Read the model definition and answer for the solid it produces. Units are mm, in the model's axes. Face numbers are marked on the shaded views. A direction names the side the tool comes from. Round coordinates to 2 decimals unless told otherwise and drop trailing zeros. Loops run counter-clockwise (first coordinate to the right, second up) from the corner with the lowest first, then second, coordinate; pieces in that order, holes last. Notation, with made-up numbers: M 89,55.5 L 130,55.5 A19 cw 130,59.5 Z; hole C -7,-27 d9. An arc over 180 degrees is marked long. Write each question's results on one line, items separated by ' | '.
```python
from build123d import *

# Parameters (mm, degrees)
CYLINDER005_R     = 1.65
CYLINDER005_DEPTH = 50
CYLINDER006_R     = 3.25
CYLINDER006_DEPTH = 2.5
BOX001_W          = 80
BOX001_H          = 100
BOX001_DEPTH      = 9.5
CYLINDER003_R     = 22.95
CYLINDER003_DEPTH = 27
CYLINDER004_R     = 27.75
CYLINDER004_DEPTH = 40
SKETCH006_R       = 27.25
SKETCH006_R_2     = 8.7
PAD_DEPTH         = 60
SKETCH007_W       = 3.5
SKETCH007_H       = 6.5
POCKET007_DEPTH   = 32.1
SKETCH008_R       = 1.7
POCKET008_DEPTH   = 30
SKETCH009_R       = 3.4
POCKET009_DEPTH   = 10
SKETCH010_R       = 1.7
POCKET010_DEPTH   = 30
SKETCH011_R       = 3.4
POCKET011_DEPTH   = 10
SKETCH012_W       = 3.5
SKETCH012_H       = 6.5
POCKET012_DEPTH   = 32.1


with BuildPart() as cylinder:
    # Cylinder005 → Cylinder005 (new body)
    with BuildSketch(Plane(origin=(0, 50, 20), x_dir=(1, 0, 0), z_dir=(0, -1, 0))):
        Circle(CYLINDER005_R)
    extrude(amount=CYLINDER005_DEPTH)


with BuildPart() as cylinder006:
    # Cylinder006 → Cylinder006 (new body)
    with BuildSketch(Plane(origin=(0, 27.75, 20), x_dir=(1, 0, 0), z_dir=(0, -1, 0))):
        Circle(CYLINDER006_R)
    extrude(amount=CYLINDER006_DEPTH)


with BuildPart() as obj1:
    # Box001 → Box001 (new body)
    with BuildSketch(Plane(origin=(-40, 0, -1), x_dir=(1, 0, 0), z_dir=(0, 0, 1))):
        with Locations((40, 50)):
            Rectangle(BOX001_W, BOX001_H)
    extrude(amount=BOX001_DEPTH)


with BuildPart() as fusion003:
    # Cylinder003 → Cylinder003 (new body)
    with BuildSketch(Plane.XY.offset(-1)):
        Circle(CYLINDER003_R)
    extrude(amount=CYLINDER003_DEPTH)

    # Cut004: cut obj1
    add(obj1.part, mode=Mode.SUBTRACT)

    # Fusion003: union Cylinder, Cylinder006
    add(cylinder.part)
    add(cylinder006.part)


with BuildPart() as obj2:
    # Cylinder004 → Cylinder004 (new body)
    with BuildSketch(Plane.XY.offset(-14)):
        Circle(CYLINDER004_R)
    extrude(amount=CYLINDER004_DEPTH)

    # Cut002: cut Fusion003
    add(fusion003.part, mode=Mode.SUBTRACT)

    # Sketch006 (on Face2 of BaseFeature002) → Pad (new body)
    with BuildSketch(Plane(origin=(0, 0, -14), x_dir=(1, 0, 0), z_dir=(0, 0, -1))):
        Circle(SKETCH006_R)
        Circle(SKETCH006_R_2, mode=Mode.SUBTRACT)
    extrude(amount=PAD_DEPTH)

    # Sketch007 → Pocket007 (cut)
    with BuildSketch(Plane.XZ.offset(28)):
        with Locations((13.75, -28.25)):
            Rectangle(SKETCH007_W, SKETCH007_H)
    extrude(amount=-POCKET007_DEPTH, mode=Mode.SUBTRACT)

    # Sketch008 → Pocket008 (cut)
    with BuildSketch(Plane.YZ.offset(28)):
        with Locations((0, -28.25)):
            Circle(SKETCH008_R)
    extrude(amount=-POCKET008_DEPTH, mode=Mode.SUBTRACT)

    # Sketch009 → Pocket009 (cut)
    with BuildSketch(Plane.YZ.offset(28)):
        with Locations((0, -28.25)):
            Circle(SKETCH009_R)
    extrude(amount=-POCKET009_DEPTH, mode=Mode.SUBTRACT)

    # Sketch010 → Pocket010 (cut)
    with BuildSketch(Plane.YZ.offset(-28)):
        with Locations((0, -28.25)):
            Circle(SKETCH010_R)
    extrude(amount=POCKET010_DEPTH, mode=Mode.SUBTRACT)

    # Sketch011 → Pocket011 (cut)
    with BuildSketch(Plane.YZ.offset(-28)):
        with Locations((0, -28.25)):
            Circle(SKETCH011_R)
    extrude(amount=POCKET011_DEPTH, mode=Mode.SUBTRACT)

    # Sketch012 → Pocket012 (cut)
    with BuildSketch(Plane(origin=(0, -28, 2), x_dir=(1, 0, 0), z_dir=(0, -1, 0))):
        with Locations((-13.75, -30.25)):
            Rectangle(SKETCH012_W, SKETCH012_H)
    extrude(amount=-POCKET012_DEPTH, mode=Mode.SUBTRACT)


solid = obj2.part
```
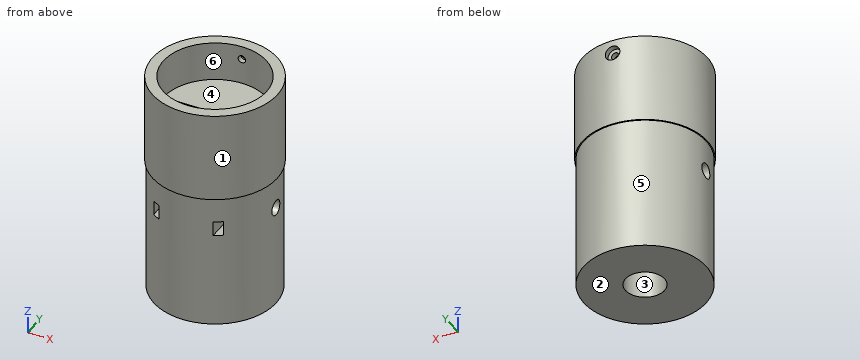
1. Find the intervals of material crossed by L1, parallel to Z at x = 0, y = 23.9; L2, parallel to Y at x = 0, z = 5; L3, parallel to Z at x = -10.5, y = -4, in increasing order.
Completed:
L1: z = -74 to 18.35, 21.65 to 26 | L2: y = -27.75 to -22.95, 0 to 27.75 | L3: z = -74 to -1
2. Determine the mould class of the marked faces 1, 2, 3 and 4 for opening direction Y: released by +Y, released by -Y, zero draft, split by the parting line, or undercut.
Completed:
face 1: split by the parting line | face 2: zero draft | face 3: undercut | face 4: undercut
3. Find section C-C, the plane y = -6. Give the vertices of the cut face in (x, z).
Completed:
outline: M -27.09,-14 L -26.58,-14 L -26.58,-74 L -6.3,-74 L -6.3,-14 L 6.3,-14 L 6.3,-74 L 26.58,-74 L 26.58,-14 L 27.09,-14 L 27.09,26 L 22.15,26 L 22.15,-1 L -22.15,-1 L -22.15,26 L -27.09,26 Z; hole M -15.5,-31.5 L -12,-31.5 L -12,-25 L -15.5,-25 Z; hole M 12,-31.5 L 15.5,-31.5 L 15.5,-25 L 12,-25 Z
4. Find section B-B, the plane z = -28.25. Count the separate pieces of the cut face and the enclosed holes in it, then the cut area to 3 significant figures.
Completed:
separate pieces: 4 | enclosed holes: 0 | area: 1,740 mm2
5. Find section D-D, the plane x = -20.5. Give the vertices of the cut face in (y, z), then the cut area to 3 significant figures.
Completed:
outline: M -18.7,-14 L -17.95,-14 L -17.95,-74 L 17.95,-74 L 17.95,-14 L 18.7,-14 L 18.7,26 L 10.32,26 L 10.32,8.5 L 0,8.5 L 0,-1 L -10.32,-1 L -10.32,26 L -18.7,26 Z; hole C 0,-28.25 d6.8 | area: 3,160 mm2
6. Which of the six approach directions +Z, -Z, +X, -X, +Y, -Y give full straight-line access (tool end or side, diameter ignored) to the marked faces 5 and 6?
Completed:
face 5: -Z | face 6: +Z
7. Given P1, Ø5.5, axis at y = 0, z = -29.5, coming from the -X side; P2, Ø10, axis at x = -22, z = -64, coming from the +Y side; P3, Ø11, axis at y = 0, z = -28.25, coming from the +X side, each flat-ended and moving along its own axis, determine where each tip first touches the part or whether it passes through.
Completed:
P1: stops at x = -27.25 | P2: stops at y = 21.3 | P3: stops at x = 27.25
8. Find section A-A, the plane x = 0. Give the vertices of the cut face in (y, z).
Completed:
outline: M -27.75,-14 L -27.25,-14 L -27.25,-74 L -8.7,-74 L -8.7,-14 L 8.7,-14 L 8.7,-74 L 27.25,-74 L 27.25,-14 L 27.75,-14 L 27.75,16.75 L 25.25,16.75 L 25.25,18.35 L 22.95,18.35 L 22.95,8.5 L 0,8.5 L 0,-1 L -22.95,-1 L -22.95,26 L -27.75,26 Z; M 22.95,21.65 L 25.25,21.65 L 25.25,23.25 L 27.75,23.25 L 27.75,26 L 22.95,26 Z
